Source: CAD feature listing. Evaluate the final solid. Frame: model axes, mm. Face numbers are marked on the shaded views. A direction names the side the tool comes from. Round coordinates to 2 decimals unless told otherwise and drop trailing zeros. Order: outer loops, then holes, each group sorted by start corner. A loop starts at its lowest first (then second) coordinate and runs counter-clockwise, first axis right, second up. Notation, with made-up numbers: (60.5, 68) -> (109.5, 68) arc R4 cw to (109.5, 73) -> close; hole circle Ø10 at (69.5, 53.5). An arc over 180 degrees is marked (long way). Answer as CSV lines item,"result".
from build123d import *

# Parameters (mm, degrees)
SKETCH2_W                 = 28
SKETCH2_H                 = 28
BOSS_EXTRUDE1_DEPTH       = 28.2
SKETCH3_R                 = 11
BOSS_EXTRUDE2_DEPTH       = 2
SKETCH4_R                 = 2.5
BOSS_EXTRUDE3_DEPTH       = 20
CUT_EXTRUDE1_DEPTH        = 18
F_2_5MM_DOWEL_HOLE1_D     = 2.5
F_2_5MM_DOWEL_HOLE1_DEPTH = 4
F_2_5MM_DOWEL_HOLE1_TIP   = 0.751075774


with BuildPart() as part:
    # Sketch2 → Boss-Extrude1 (new body)
    with BuildSketch(Plane.XY):
        Rectangle(SKETCH2_W, SKETCH2_H)
    extrude(amount=-BOSS_EXTRUDE1_DEPTH)

    # Sketch3 → Boss-Extrude2 (add)
    with BuildSketch(Plane.XY):
        Circle(SKETCH3_R)
    extrude(amount=BOSS_EXTRUDE2_DEPTH)

    # Sketch4 → Boss-Extrude3 (add)
    with BuildSketch(Plane.XY):
        Circle(SKETCH4_R)
    extrude(amount=BOSS_EXTRUDE3_DEPTH)

    # Sketch5 → Cut-Extrude1 (cut)
    with BuildSketch(Plane.XY.offset(20)):
        Polygon((2, 56.05333882), (2, 1.5), (2, -1.5), (2, -56.05333882), (111.10667764, -56.05333882), (111.10667764, 56.05333882), align=None)
    extrude(amount=-CUT_EXTRUDE1_DEPTH, mode=Mode.SUBTRACT)

    # Ø2.5mm Dowel Hole1
    with Locations(Plane.XY):
        with Locations((-11.325, 11.325), (11.325, 11.325), (11.325, -11.325), (-11.325, -11.325)):
            Hole(F_2_5MM_DOWEL_HOLE1_D / 2, depth=F_2_5MM_DOWEL_HOLE1_DEPTH)
            with Locations((0, 0, -(F_2_5MM_DOWEL_HOLE1_DEPTH + F_2_5MM_DOWEL_HOLE1_TIP / 2))):  # 118° drill point
                Cone(0, F_2_5MM_DOWEL_HOLE1_D / 2, F_2_5MM_DOWEL_HOLE1_TIP, mode=Mode.SUBTRACT)


solid = part.part
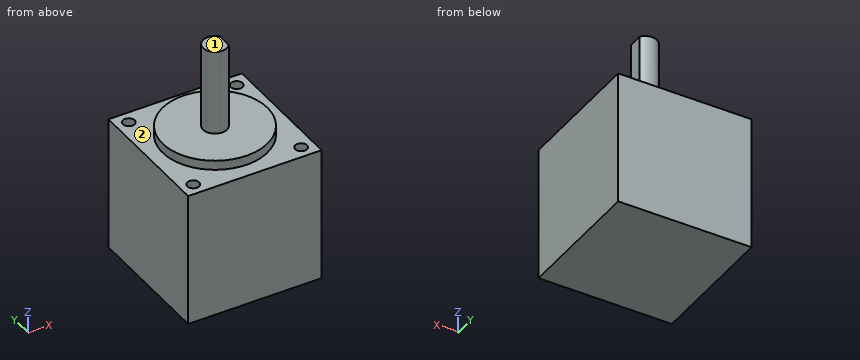
1. Line query: L1, parallel to Z at x = 3, y = 9.75; L2, parallel to Z at x = 12.5, y = 0.5; L3, parallel to X at y = -2, z = 13. Output: solid intervals per line, ascending. Write a range as [from, to].
Results below:
L1,"[-28.2, 2]"
L2,"[-28.2, 0]"
L3,"[-1.5, 1.5]"
2. Section query A-A on y = 0. Return loops of the section in (x, z), and give its area (3 significant figures).
Results below:
outline,"(-14, -28.2) -> (14, -28.2) -> (14, 0) -> (11, 0) -> (11, 2) -> (2, 2) -> (2, 20) -> (-2.5, 20) -> (-2.5, 2) -> (-11, 2) -> (-11, 0) -> (-14, 0) -> close"
area,"915 mm2"
3. Pin query (flat end, axial travel): pin 1 (3.5 mm diameter, centred on y = 0.5, z = 14, fed in from +X); pin 2 (8 mm diameter, centred on y = 9.5, z = 9, fed in from +X); pin 3 (2 mm diameter, centred on x = -11.325, y = -11.325, fed in from +Z). Return the tip coordinate at first contact, or that it passes through.
Results below:
pin 1,"x = 2"
pin 2,"through"
pin 3,"z = -4.15"
4. Section query C-C on z = 3.5. Return loops of the section in (x, y), and give its area (3 significant figures).
Results below:
outline,"(2, -1.5) -> (2, 1.5) arc R2.5 ccw (long way) to start"
area,"18.6 mm2"
5. Section query B-B on x = 0. Return loops of the section in (y, z).
Results below:
outline,"(-14, -28.2) -> (14, -28.2) -> (14, 0) -> (11, 0) -> (11, 2) -> (2.5, 2) -> (2.5, 20) -> (-2.5, 20) -> (-2.5, 2) -> (-11, 2) -> (-11, 0) -> (-14, 0) -> close"
6. Section query D-D on y = 6. Return loops of the section in (x, z), and give its area (3 significant figures).
Results below:
outline,"(-14, -28.2) -> (14, -28.2) -> (14, 0) -> (9.22, 0) -> (9.22, 2) -> (-9.22, 2) -> (-9.22, 0) -> (-14, 0) -> close"
area,"826 mm2"
7. Reachability of the marked faces 1 and 2 from +Z, -Z, +X, -X, +Y, -Y: full face, straight path, thin tool, end or side. Return the list, or none.
Results below:
face 1,"+Z, +X, -X, +Y, -Y"
face 2,"+Z"
